```python
from build123d import *

# Parameters (mm, degrees)
ESQUISSE1_R             = 46.46108
BOSS_EXTRU_1_DEPTH      = 10
ESQUISSE2_R             = 29.44481
ENL_V_MAT_EXTRU_1_DEPTH = 67.462500025
ESQUISSE4_W             = 0.6
ESQUISSE4_H             = 40
ESQUISSE4_W_2           = 40
ESQUISSE4_H_2           = 0.6
ENL_V_MAT_EXTRU_2_DEPTH = 10
ESQUISSE5_R             = 29.44481
BOSS_EXTRU_2_DEPTH      = 10
ESQUISSE6_R             = 28.94481
ENL_V_MAT_EXTRU_3_DEPTH = 67.461145864
ESQUISSE7_R             = 47.46108
ESQUISSE7_R_2           = 46.46108
BOSS_EXTRU_3_DEPTH      = 10


with BuildPart() as part:
    # Esquisse1 → Boss.-Extru.1 (new body)
    with BuildSketch(Plane.XY):
        Circle(ESQUISSE1_R)
    extrude(amount=BOSS_EXTRU_1_DEPTH)

    # Esquisse2 → Enl_v. mat.-Extru.1 (cut, through all)
    with BuildSketch(Plane.XY.offset(10)):
        Circle(ESQUISSE2_R)
    extrude(amount=-ENL_V_MAT_EXTRU_1_DEPTH, mode=Mode.SUBTRACT)

    # Esquisse4 → Enl_v. mat.-Extru.2 (cut)
    with BuildSketch(Plane.XY.offset(10)):
        Polygon((23.238169802, 55.317966921), (7.930832507, 18.362785621), (7.376504788, 18.59239568), (22.683842082, 55.54757698), align=None)
        with Locations((0, 40)):
            Rectangle(ESQUISSE4_W, ESQUISSE4_H)
        Polygon((42.638538906, 42.214274837), (14.354267658, 13.930003589), (13.930003589, 14.354267658), (42.214274837, 42.638538906), align=None)
        Polygon((55.54757698, 22.683842082), (18.59239568, 7.376504788), (18.362785621, 7.930832507), (55.317966921, 23.238169802), align=None)
        with Locations((40, 0)):
            Rectangle(ESQUISSE4_W_2, ESQUISSE4_H_2)
        Polygon((55.317966921, -23.238169802), (18.362785621, -7.930832507), (18.59239568, -7.376504788), (55.54757698, -22.683842082), align=None)
        Polygon((42.214274837, -42.638538906), (13.930003589, -14.354267658), (14.354267658, -13.930003589), (42.638538906, -42.214274837), align=None)
        Polygon((22.683842082, -55.54757698), (7.376504788, -18.59239568), (7.930832507, -18.362785621), (23.238169802, -55.317966921), align=None)
        with Locations((0, -40)):
            Rectangle(ESQUISSE4_W, ESQUISSE4_H)
        Polygon((-23.238169802, -55.317966921), (-7.930832507, -18.362785621), (-7.376504788, -18.59239568), (-22.683842082, -55.54757698), align=None)
        Polygon((-42.638538906, -42.214274837), (-14.354267658, -13.930003589), (-13.930003589, -14.354267658), (-42.214274837, -42.638538906), align=None)
        Polygon((-55.54757698, -22.683842082), (-18.59239568, -7.376504788), (-18.362785621, -7.930832507), (-55.317966921, -23.238169802), align=None)
        with Locations((-40, 0)):
            Rectangle(ESQUISSE4_W_2, ESQUISSE4_H_2)
        Polygon((-55.317966921, 23.238169802), (-18.362785621, 7.930832507), (-18.59239568, 7.376504788), (-55.54757698, 22.683842082), align=None)
        Polygon((-42.214274837, 42.638538906), (-13.930003589, 14.354267658), (-14.354267658, 13.930003589), (-42.638538906, 42.214274837), align=None)
        Polygon((-22.683842082, 55.54757698), (-7.376504788, 18.59239568), (-7.930832507, 18.362785621), (-23.238169802, 55.317966921), align=None)
    extrude(amount=-ENL_V_MAT_EXTRU_2_DEPTH, mode=Mode.SUBTRACT)


with BuildPart() as enl_v_mat_extru_2_piece_1:
    # of the separate pieces the step leaves, piece 1, a body of its own (enl_v_mat_extru_2_pieces)
    add(part.part.solids().sort_by_distance((-32.640127818, -33.064391886, 0))[0])



with BuildPart() as enl_v_mat_extru_2_piece_2:
    # of the separate pieces the step leaves, piece 2, a body of its own (enl_v_mat_extru_2_pieces)
    add(part.part.solids().sort_by_distance((-18.056678773, 42.808741005, 0))[0])


with BuildPart() as enl_v_mat_extru_2_piece_3:
    # of the separate pieces the step leaves, piece 3, a body of its own (enl_v_mat_extru_2_pieces)
    add(part.part.solids().sort_by_distance((-42.808741005, -18.056678773, 0))[0])


with BuildPart() as enl_v_mat_extru_2_piece_4:
    # of the separate pieces the step leaves, piece 4, a body of its own (enl_v_mat_extru_2_pieces)
    add(part.part.solids().sort_by_distance((-33.064391886, 32.640127818, 0))[0])


with BuildPart() as enl_v_mat_extru_2_piece_5:
    # of the separate pieces the step leaves, piece 5, a body of its own (enl_v_mat_extru_2_pieces)
    add(part.part.solids().sort_by_distance((17.502351053, 43.038351065, 0))[0])


with BuildPart() as enl_v_mat_extru_2_piece_6:
    # of the separate pieces the step leaves, piece 6, a body of its own (enl_v_mat_extru_2_pieces)
    add(part.part.solids().sort_by_distance((0.3, -46.460111437, 0))[0])


with BuildPart() as enl_v_mat_extru_2_piece_7:
    # of the separate pieces the step leaves, piece 7, a body of its own (enl_v_mat_extru_2_pieces)
    add(part.part.solids().sort_by_distance((-0.3, 46.460111437, 0))[0])


with BuildPart() as enl_v_mat_extru_2_piece_8:
    # of the separate pieces the step leaves, piece 8, a body of its own (enl_v_mat_extru_2_pieces)
    add(part.part.solids().sort_by_distance((46.460111437, 0.3, 0))[0])


with BuildPart() as enl_v_mat_extru_2_piece_9:
    # of the separate pieces the step leaves, piece 9, a body of its own (enl_v_mat_extru_2_pieces)
    add(part.part.solids().sort_by_distance((43.038351065, -17.502351053, 0))[0])


with BuildPart() as enl_v_mat_extru_2_piece_10:
    # of the separate pieces the step leaves, piece 10, a body of its own (enl_v_mat_extru_2_pieces)
    add(part.part.solids().sort_by_distance((-17.502351053, -43.038351065, 0))[0])


with BuildPart() as enl_v_mat_extru_2_piece_11:
    # of the separate pieces the step leaves, piece 11, a body of its own (enl_v_mat_extru_2_pieces)
    add(part.part.solids().sort_by_distance((32.640127818, 33.064391886, 0))[0])


with BuildPart() as enl_v_mat_extru_2_piece_12:
    # of the separate pieces the step leaves, piece 12, a body of its own (enl_v_mat_extru_2_pieces)
    add(part.part.solids().sort_by_distance((42.808741005, 18.056678773, 0))[0])


with BuildPart() as enl_v_mat_extru_2_piece_13:
    # of the separate pieces the step leaves, piece 13, a body of its own (enl_v_mat_extru_2_pieces)
    add(part.part.solids().sort_by_distance((18.056678773, -42.808741005, 0))[0])


with BuildPart() as enl_v_mat_extru_2_piece_14:
    # of the separate pieces the step leaves, piece 14, a body of its own (enl_v_mat_extru_2_pieces)
    add(part.part.solids().sort_by_distance((33.064391886, -32.640127818, 0))[0])


with BuildPart() as enl_v_mat_extru_2_piece_15:
    # of the separate pieces the step leaves, piece 15, a body of its own (enl_v_mat_extru_2_pieces)
    add(part.part.solids().sort_by_distance((-46.460111437, -0.3, 0))[0])


with BuildPart() as enl_v_mat_extru_2_piece_16:
    # of the separate pieces the step leaves, piece 16, a body of its own (enl_v_mat_extru_2_pieces)
    add(part.part.solids().sort_by_distance((-43.038351065, 17.502351053, 0))[0])


with BuildPart() as enl_v_mat_extru_2_piece_1_1:
    add(enl_v_mat_extru_2_piece_1.part)

    add(enl_v_mat_extru_2_piece_2.part)  # Boss.-Extru.2 merges Enl_v. mat.-Extru.2 piece 2

    add(enl_v_mat_extru_2_piece_3.part)  # Boss.-Extru.2 merges Enl_v. mat.-Extru.2 piece 3

    add(enl_v_mat_extru_2_piece_4.part)  # Boss.-Extru.2 merges Enl_v. mat.-Extru.2 piece 4

    add(enl_v_mat_extru_2_piece_5.part)  # Boss.-Extru.2 merges Enl_v. mat.-Extru.2 piece 5

    add(enl_v_mat_extru_2_piece_6.part)  # Boss.-Extru.2 merges Enl_v. mat.-Extru.2 piece 6

    add(enl_v_mat_extru_2_piece_7.part)  # Boss.-Extru.2 merges Enl_v. mat.-Extru.2 piece 7

    add(enl_v_mat_extru_2_piece_8.part)  # Boss.-Extru.2 merges Enl_v. mat.-Extru.2 piece 8

    add(enl_v_mat_extru_2_piece_9.part)  # Boss.-Extru.2 merges Enl_v. mat.-Extru.2 piece 9

    add(enl_v_mat_extru_2_piece_10.part)  # Boss.-Extru.2 merges Enl_v. mat.-Extru.2 piece 10

    add(enl_v_mat_extru_2_piece_11.part)  # Boss.-Extru.2 merges Enl_v. mat.-Extru.2 piece 11

    add(enl_v_mat_extru_2_piece_12.part)  # Boss.-Extru.2 merges Enl_v. mat.-Extru.2 piece 12

    add(enl_v_mat_extru_2_piece_13.part)  # Boss.-Extru.2 merges Enl_v. mat.-Extru.2 piece 13

    add(enl_v_mat_extru_2_piece_14.part)  # Boss.-Extru.2 merges Enl_v. mat.-Extru.2 piece 14

    add(enl_v_mat_extru_2_piece_15.part)  # Boss.-Extru.2 merges Enl_v. mat.-Extru.2 piece 15

    add(enl_v_mat_extru_2_piece_16.part)  # Boss.-Extru.2 merges Enl_v. mat.-Extru.2 piece 16
    # Esquisse5 → Boss.-Extru.2 (add)
    with BuildSketch(Plane.XY):
        Circle(ESQUISSE5_R)
    extrude(amount=BOSS_EXTRU_2_DEPTH)

    # Esquisse6 → Enl_v. mat.-Extru.3 (cut, through all)
    with BuildSketch(Plane.XY.offset(10)):
        Circle(ESQUISSE6_R)
    extrude(amount=-ENL_V_MAT_EXTRU_3_DEPTH, mode=Mode.SUBTRACT)

    # Esquisse7 → Boss.-Extru.3 (add)
    with BuildSketch(Plane.XY):
        Circle(ESQUISSE7_R)
        Circle(ESQUISSE7_R_2, mode=Mode.SUBTRACT)
    extrude(amount=BOSS_EXTRU_3_DEPTH)


solid = enl_v_mat_extru_2_piece_1_1.part
```
Build history of the part. All positions in model axes, mm. Round coordinates to 2 decimals unless told otherwise and drop trailing zeros. Write each loop counter-clockwise with the first axis right and the second up, starting at its lowest first coordinate (ties: lowest second). Pieces come first, ordered by that corner, then holes. Notation, with made-up numbers: (71.5, 0.5) -> (126.5, 0.5) arc R15 cw to (126.5, 10.5) -> close; hole circle Ø7 at (-15.5, 42). An arc over 180 degrees is marked (long way). Put each result on its own line as item: value.
Item 1: Slice it at A-A, the plane y = 8. Give the cut face in (x, z).
Here are the results:
outline: (-46.78, 0) -> (-27.82, 0) -> (-27.82, 10) -> (-46.78, 10) -> close; (27.82, 0) -> (46.78, 0) -> (46.78, 10) -> (27.82, 10) -> close
Item 2: Slice it at C-C, the plane x = 22.5. Give the cut face in (y, z), plus the area to 3 significant figures.
Here are the results:
outline: (-41.79, 0) -> (-22.92, 0) -> (-22.92, 10) -> (-41.79, 10) -> close; (-22.08, 0) -> (-18.21, 0) -> (-18.21, 10) -> (-22.08, 10) -> close; (18.21, 0) -> (22.08, 0) -> (22.08, 10) -> (18.21, 10) -> close; (22.92, 0) -> (41.79, 0) -> (41.79, 10) -> (22.92, 10) -> close
area: 455 mm^2
Item 3: Two-plate mould, pull along Y, no slides. Class faces 1 (the face through (26.964, -26.54, 5.07)), 2 (the face through (-10.289, -46.332, 4.93)), 3 (the face through (-1, -31, 0)), 4 (the face through (26.708, -27.132, 5.07)): pulls with the +Y half, pulls with the -Y half, needs draft (parallel to the pull), parting line crosses it, or undercut.
Here are the results:
face 1: undercut
face 2: parting line crosses it
face 3: needs draft
face 4: undercut
Item 4: Slice it at D-D, the plane z = 3. Count the separate pieces of the cut face and the enclosed holes in it, plus the area to 3 significant figures.
Here are the results:
separate pieces: 1
enclosed holes: 17
area: 4,280 mm^2
Item 5: Slice it at B-B, the plane x = 7. Give the cut face in (y, z).
Here are the results:
outline: (-46.94, 0) -> (-28.09, 0) -> (-28.09, 10) -> (-46.94, 10) -> close; (28.09, 0) -> (46.94, 0) -> (46.94, 10) -> (28.09, 10) -> close
Item 6: Flat gauge pins, fed straight in: P1, Ø5, axis at x = 3, z = 2, coming from the +Y side; P2, Ø3, axis at y = 37, z = 6, coming from the +X side; P3, Ø5, axis at x = -40.5, z = 3.5, coming from the +Y side. Where does each tip first touch, or does it go through?
Here are the results:
P1: stops at y = 47.46
P2: stops at x = 31.5
P3: stops at y = 28.44
Item 7: Wall check: probe 1 along Y at (x, z) = (0, 5.25); probe 2 along Y at (x, z) = (14.5, 1.25); probe 3 along X at (y, z) = (37.5, 1.75). Give the ranges that are in metal, low to high. Write a range as from..to.
Here are the results:
probe 1: y = -47.46..-46.46, -29.44..-28.94, 28.94..29.44, 46.46..47.46
probe 2: y = -45.19..-35.79, -34.22..-25.05, 25.05..34.22, 35.79..45.19
probe 3: x = -29.09..-15.86, -15.21..-0.3, 0.3..15.21, 15.86..29.09
